```python
from build123d import *

# Parameters (mm, degrees)
BOSS_EXTRUDE1_DEPTH        = 25
BOSS_EXTRUDE1_DEPTH_BACK   = 25
BOSS_EXTRUDE1_2_DEPTH      = 25
BOSS_EXTRUDE1_2_DEPTH_BACK = 25
BOSS_EXTRUDE2_REACH        = 114.472
SKETCH3_W                  = 30
SKETCH3_H                  = 40
CUT_EXTRUDE1_DEPTH         = 89.600225733
HOLE1_D                    = 15


with BuildPart() as part:
    # Sketch1 → Boss-Extrude1 (new, two sides: drawn at the far end of the back side and taken through both)
    with BuildSketch(Plane.XY.offset(-BOSS_EXTRUDE1_DEPTH_BACK)):
        with BuildLine():
            Line((-35, 30), (-35, -30))
            ThreePointArc((-35, -30), (-50, -45), (-65, -30))
            Line((-65, -30), (-65, 30))
            ThreePointArc((-65, 30), (-50, 45), (-35, 30))
        make_face()
        with BuildLine():
            Line((-40, 30), (-40, -30))
            ThreePointArc((-40, -30), (-50, -40), (-60, -30))
            Line((-60, -30), (-60, 30))
            ThreePointArc((-60, 30), (-50, 40), (-40, 30))
        make_face(mode=Mode.SUBTRACT)
    extrude(amount=BOSS_EXTRUDE1_DEPTH + BOSS_EXTRUDE1_DEPTH_BACK)


with BuildPart() as body_2:
    # Sketch1 → Boss-Extrude1 2 (new, two sides: drawn at the far end of the back side and taken through both)
    with BuildSketch(Plane.XY.offset(-BOSS_EXTRUDE1_2_DEPTH_BACK)):
        with BuildLine():
            Line((35, 30), (35, -30))
            ThreePointArc((35, -30), (50, -45), (65, -30))
            Line((65, -30), (65, 30))
            ThreePointArc((65, 30), (50, 45), (35, 30))
        make_face()
        with BuildLine():
            Line((40, 30), (40, -30))
            ThreePointArc((40, -30), (50, -40), (60, -30))
            Line((60, -30), (60, 30))
            ThreePointArc((60, 30), (50, 40), (40, 30))
        make_face(mode=Mode.SUBTRACT)
    extrude(amount=BOSS_EXTRUDE1_2_DEPTH + BOSS_EXTRUDE1_2_DEPTH_BACK)

    # Sketch3 → Boss-Extrude2 (add, up to next)
    with BuildSketch(Plane(origin=(-35, 0, 0), x_dir=(0, 0, -1), z_dir=(1, 0, 0)), mode=Mode.PRIVATE) as boss_extrude2_sk1:
        Rectangle(SKETCH3_W, SKETCH3_H)
    boss_extrude2_tool1 = extrude(boss_extrude2_sk1.sketch, amount=BOSS_EXTRUDE2_REACH, mode=Mode.PRIVATE) - body_2.part

    add(part.part)  # Boss-Extrude2 merges part
    add(boss_extrude2_tool1.solids().sort_by_distance((-35, 0, 0))[0])

    # Sketch4 → Cut-Extrude1 (cut, through all)
    with BuildSketch(Plane(origin=(0, 0, -15), x_dir=(-1, 0, 0), z_dir=(0, 0, -1))):
        with BuildLine():
            Line((-20, 10), (20, 10))
            ThreePointArc((20, 10), (30, 0), (20, -10))
            Line((20, -10), (-20, -10))
            ThreePointArc((-20, -10), (-30, 0), (-20, 10))
        make_face()
    extrude(amount=-CUT_EXTRUDE1_DEPTH, mode=Mode.SUBTRACT)

    # Hole1 (through all)
    with Locations(Plane(origin=(65, 0, 0), x_dir=(0, 0, -1), z_dir=(1, 0, 0))):
        with Locations((0, 0)):
            Hole(HOLE1_D / 2)


solid = body_2.part
```
Can you work these out from the model? Positions are in its coordinate system, mm. A direction names the side the tool comes from. Coordinates: 2 decimals unless noted, no trailing zeros. Loops run counter-clockwise (first coordinate to the right, second up) from the corner with the lowest first, then second, coordinate; pieces in that order, holes last. Notation, with made-up numbers: (-12, 73.25) - (35, 73.25) arc R19 cw to (35, 81.25) - close; hole circle Ø1 at (-9, 82.5). An arc over 180 degrees is marked (long way). Use a Markdown table: item, result.
Item 1: Will these pins go through, and if not, where does the flat tip stop? pin 1 (1.5 mm diameter, centred on x = 13.5, z = -14, fed in from +Y); pin 2 (9 mm diameter, centred on x = -16, z = 1, fed in from -Y); pin 3 (20 mm diameter, centred on x = 11.5, y = 7.5, fed in from +Z).
Numbers:
| item | result |
|---|---|
| pin 1 | stops at y = 20 |
| pin 2 | stops at y = -20 |
| pin 3 | stops at z = 15 |
Item 2: I want a section at A-A on z = -19. Please give me the cut outline in (x, y).
Numbers:
| item | result |
|---|---|
| outline | (-65, -30) arc R15 ccw to (-35, -30) - (-35, 30) arc R15 ccw to (-65, 30) - close; (35, -30) arc R15 ccw to (65, -30) - (65, 30) arc R15 ccw to (35, 30) - close; hole (-60, -30) arc R10 ccw to (-40, -30) - (-40, 30) arc R10 ccw to (-60, 30) - close; hole (40, -30) arc R10 ccw to (60, -30) - (60, 30) arc R10 ccw to (40, 30) - close |
Item 3: We'd pull the mould along Z, two halves only. Please class faces 1 (the face through (-62.535, 0.33, -7.493)), 2 (the face through (39.8, 0.6, 25)), 3 (the face through (-50, 40, 0)): released by +Z, released by -Z, zero draft, split by the parting line, or undercut.
Numbers:
| item | result |
|---|---|
| face 1 | undercut |
| face 2 | released by +Z |
| face 3 | zero draft |
Item 4: For faces 4 (the face through (-40, 7, -6)), 5 (the face through (39.8, 0.6, -25)), 6 (the face through (0, -14, 15)), which set-ups out of +Z, -Z, +X, -X, +Y, -Y let a thin tool reach every point of the face, with its end or its side?
Numbers:
| item | result |
|---|---|
| face 4 | +Z, -Z |
| face 5 | -Z, +X, -X, +Y, -Y |
| face 6 | +Z, +Y, -Y |
Item 5: I want a section at D-D on z = 11.5. Please give me the cut outline in (x, y).
Numbers:
| item | result |
|---|---|
| outline | (-65, -30) arc R15 ccw to (-35, -30) - (-35, -20) - (35, -20) - (35, -30) arc R15 ccw to (65, -30) - (65, 30) arc R15 ccw to (35, 30) - (35, 20) - (-35, 20) - (-35, 30) arc R15 ccw to (-65, 30) - close; hole (-60, -30) arc R10 ccw to (-40, -30) - (-40, 30) arc R10 ccw to (-60, 30) - close; hole (-20, -10) - (20, -10) arc R10 ccw to (20, 10) - (-20, 10) arc R10 ccw to start; hole (40, -30) arc R10 ccw to (60, -30) - (60, 30) arc R10 ccw to (40, 30) - close |
Item 6: I want a section at B-B on y = -21.5. Please give me the cut outline in (x, z), and give its area (3 significant figures).
Numbers:
| item | result |
|---|---|
| outline | (-65, -25) - (-60, -25) - (-60, 25) - (-65, 25) - close; (-40, -25) - (-35, -25) - (-35, 25) - (-40, 25) - close; (35, -25) - (40, -25) - (40, 25) - (35, 25) - close; (60, -25) - (65, -25) - (65, 25) - (60, 25) - close |
| area | 1,000 mm2 |
Item 7: I want a section at C-C on x = -50. Please give me the cut outline in (y, z), and give its area (3 significant figures).
Numbers:
| item | result |
|---|---|
| outline | (-45, -25) - (-40, -25) - (-40, 25) - (-45, 25) - close; (40, -25) - (45, -25) - (45, 25) - (40, 25) - close |
| area | 500 mm2 |
Item 8: If I drill on probe 1 along X at (y, z) = (-30, 22); probe 2 along X at (y, z) = (-18, -6); probe 3 along Y at (x, z) = (-32, 0), over which ranges is the centre line in solid material (lowest first)? Write a range as from..to.
Numbers:
| item | result |
|---|---|
| probe 1 | x = -65..-60, -40..-35, 35..40, 60..65 |
| probe 2 | x = -65..-60, -40..40, 60..65 |
| probe 3 | y = -20..-7.5, 7.5..20 |
